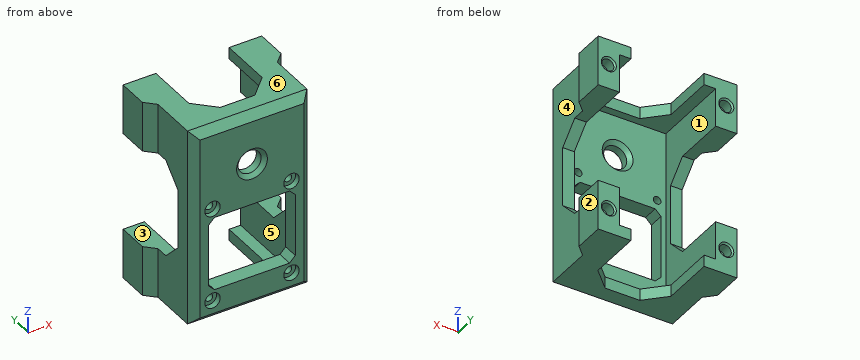
```python
from build123d import *

# Parameters (mm, degrees)
SKETCH1_W                                  = 25
SKETCH1_H                                  = 45.5
BOSS_EXTRUDE1_DEPTH                        = 4
SKETCH2_R                                  = 1
CUT_EXTRUDE1_DEPTH                         = 27.264281829
SKETCH3_W                                  = 22.5
SKETCH3_H                                  = 19.25
CUT_EXTRUDE2_DEPTH                         = 4
CHAMFER1_SIZE                              = 1.5
SKETCH4_R                                  = 3
CUT_EXTRUDE3_DEPTH                         = 27.264281829
SKETCH11_W                                 = 31
SKETCH11_H                                 = 51.5
SKETCH11_W_2                               = 25
SKETCH11_H_2                               = 45.5
BOSS_EXTRUDE5_DEPTH                        = 6
BOSS_EXTRUDE6_DEPTH                        = 18.75
SKETCH14_W                                 = 5.5
SKETCH14_H                                 = 13
BOSS_EXTRUDE7_DEPTH                        = 8
SKETCH15_R                                 = 1.55
CUT_EXTRUDE5_DEPTH                         = 3
MIRROR2_AT_THE_SECOND_PLANE_COPY_1_DEPTH   = 18.75
MIRROR2_AT_THE_SECOND_PLANE_COPY_2_SKETC_W = 5.5
MIRROR2_AT_THE_SECOND_PLANE_COPY_2_SKETC_H = 13
MIRROR2_AT_THE_SECOND_PLANE_COPY_2_DEPTH   = 8
MIRROR2_AT_THE_SECOND_PLANE_COPY_3_SKETC_R = 1.55
MIRROR2_AT_THE_SECOND_PLANE_COPY_3_DEPTH   = 3
CHAMFER3_SIZE                              = 2.5
CHAMFER4_SIZE                              = 5
CHAMFER5_SIZE                              = 2
SKETCH16_R                                 = 2
CUT_EXTRUDE6_DEPTH                         = 1.5
CHAMFER6_SIZE                              = 1
CHAMFER7_SIZE                              = 0.4
SKETCH17_R                                 = 1
CUT_EXTRUDE7_DEPTH                         = 4


with BuildPart() as part:
    # Sketch1 → Boss-Extrude1 (new body)
    with BuildSketch(Plane(origin=(0, 0, 0), x_dir=(1, 0, 0), z_dir=(0, 1, 0))):
        Rectangle(SKETCH1_W, SKETCH1_H)
    extrude(amount=BOSS_EXTRUDE1_DEPTH)

    # Sketch2 → Cut-Extrude1 (cut, through all)
    with BuildSketch(Plane(origin=(0, 4, 0), x_dir=(1, 0, 0), z_dir=(0, 1, 0))):
        with Locations(Location((-10.25, 20.25, 0), (0, 0, 270))):
            Circle(SKETCH2_R)
        with Locations(Location((10.25, 20.25, 0), (0, 0, 270))):
            Circle(SKETCH2_R)
        with Locations(Location((10.25, -4.2, 0), (0, 0, 270))):
            Circle(SKETCH2_R)
        with Locations(Location((-10.25, -4.2, 0), (0, 0, 270))):
            Circle(SKETCH2_R)
    extrude(amount=-CUT_EXTRUDE1_DEPTH, mode=Mode.SUBTRACT)

    # Sketch3 → Cut-Extrude2 (cut)
    with BuildSketch(Plane(origin=(0, 4, 0), x_dir=(1, 0, 0), z_dir=(0, 1, 0))):
        with Locations((0, 7.875)):
            Rectangle(SKETCH3_W, SKETCH3_H)
    extrude(amount=-CUT_EXTRUDE2_DEPTH, mode=Mode.SUBTRACT)

    # Chamfer1
    chamfer1_edges = [part.edges().sort_by_distance(p)[0] for p in [
        (11.25, 2, -17.5),
        (11.25, 2, 1.75),
        (-11.25, 2, 1.75),
        (-11.25, 2, -17.5),
    ]]
    chamfer(chamfer1_edges, length=CHAMFER1_SIZE)

    # Sketch4 → Cut-Extrude3 (cut, through all)
    with BuildSketch(Plane(origin=(0, 4, 0), x_dir=(1, 0, 0), z_dir=(0, 1, 0))):
        with Locations(Location((0, -12.5, 0), (0, 0, 270))):
            Circle(SKETCH4_R)
    extrude(amount=-CUT_EXTRUDE3_DEPTH, mode=Mode.SUBTRACT)

    # Sketch11 → Boss-Extrude5 (add)
    with BuildSketch(Plane.XZ):
        Rectangle(SKETCH11_W, SKETCH11_H)
        Rectangle(SKETCH11_W_2, SKETCH11_H_2, mode=Mode.SUBTRACT)
    extrude(amount=-BOSS_EXTRUDE5_DEPTH)

    # Sketch12 → Boss-Extrude6 (add)
    with BuildSketch(Plane(origin=(0, 6, 0), x_dir=(1, 0, 0), z_dir=(0, 1, 0))):
        Polygon((-15.5, 25.75), (-9.5, 25.75), (-9.5, 22.75), (-12.5, 22.75), (-12.5, 12.75), (-15.5, 12.75), align=None)
    boss_extrude6 = extrude(amount=BOSS_EXTRUDE6_DEPTH)

    # Sketch14 → Boss-Extrude7 (add)
    with BuildSketch(Plane(origin=(0, 24.75, 0), x_dir=(1, 0, 0), z_dir=(0, 1, 0))):
        with Locations((-15.25, 19.25)):
            Rectangle(SKETCH14_W, SKETCH14_H)
    boss_extrude7 = extrude(amount=-BOSS_EXTRUDE7_DEPTH)

    # Sketch15 → Cut-Extrude5 (cut)
    with BuildSketch(Plane(origin=(0, 24.75, 0), x_dir=(1, 0, 0), z_dir=(0, 1, 0))):
        with Locations(Location((-15.25, 19.25, 0), (0, 0, 270))):
            Circle(SKETCH15_R)
    cut_extrude5 = extrude(amount=-CUT_EXTRUDE5_DEPTH, mode=Mode.SUBTRACT)

    # Mirror2: Boss-Extrude6, Boss-Extrude7, Cut-Extrude5 across plane
    add(boss_extrude6.mirror(Plane(origin=(0, 0, 0), x_dir=(0, 0, 1), z_dir=(1, 0, 0))))
    add(boss_extrude7.mirror(Plane(origin=(0, 0, 0), x_dir=(0, 0, 1), z_dir=(1, 0, 0))))
    add(cut_extrude5.mirror(Plane(origin=(0, 0, 0), x_dir=(0, 0, 1), z_dir=(1, 0, 0))), mode=Mode.SUBTRACT)

    # Mirror2 at the second plane: Boss-Extrude6, Boss-Extrude7, Cut-Extrude5 across plane
    add(boss_extrude6.mirror(Plane.XY))
    add(boss_extrude7.mirror(Plane.XY))
    add(cut_extrude5.mirror(Plane.XY), mode=Mode.SUBTRACT)

    # Mirror2 at the second plane copy 1 sketc → Mirror2 at the second plane copy 1 (add)
    with BuildSketch(Plane(origin=(0, 6, 0), x_dir=(-1, 0, 0), z_dir=(0, 1, 0))):
        Polygon((-15.5, 25.75), (-9.5, 25.75), (-9.5, 22.75), (-12.5, 22.75), (-12.5, 12.75), (-15.5, 12.75), align=None)
    extrude(amount=MIRROR2_AT_THE_SECOND_PLANE_COPY_1_DEPTH)

    # Mirror2 at the second plane copy 2 sketc → Mirror2 at the second plane copy 2 (add)
    with BuildSketch(Plane(origin=(0, 24.75, 0), x_dir=(-1, 0, 0), z_dir=(0, 1, 0))):
        with Locations((-15.25, 19.25)):
            Rectangle(MIRROR2_AT_THE_SECOND_PLANE_COPY_2_SKETC_W, MIRROR2_AT_THE_SECOND_PLANE_COPY_2_SKETC_H)
    extrude(amount=-MIRROR2_AT_THE_SECOND_PLANE_COPY_2_DEPTH)

    # Mirror2 at the second plane copy 3 sketc → Mirror2 at the second plane copy 3 (cut)
    with BuildSketch(Plane(origin=(0, 24.75, 0), x_dir=(-1, 0, 0), z_dir=(0, 1, 0))):
        with Locations(Location((-15.25, 19.25, 0), (0, 0, 270))):
            Circle(MIRROR2_AT_THE_SECOND_PLANE_COPY_3_SKETC_R)
    extrude(amount=-MIRROR2_AT_THE_SECOND_PLANE_COPY_3_DEPTH, mode=Mode.SUBTRACT)

    # Chamfer3
    # the kernel refuses this chamfer: 2.5 mm, written as the material it adds along each edge
    with BuildSketch(Plane(origin=(-15.5, 16.75, -12.75), x_dir=(0.027495876610586317, -0.9996219169112968, 0), z_dir=(0, 0, -1))) as chamfer3_piece_1_section:
        Polygon((CHAMFER3_SIZE * 0.999621916911, CHAMFER3_SIZE * 0.0274958766106), (-CHAMFER3_SIZE * 0.0274958766106, CHAMFER3_SIZE * 0.999621916911), (0, 0), align=None)
    chamfer3_piece_1 = extrude(amount=13, mode=Mode.PRIVATE)
    chamfer3_piece_1 = split(chamfer3_piece_1, bisect_by=Plane(origin=(-18, 15.923989614, -19.25), z_dir=(1, 0, 0)), keep=Keep.TOP, mode=Mode.PRIVATE)
    add(chamfer3_piece_1)
    with BuildSketch(Plane(origin=(-15.5, 16.75, 12.75), x_dir=(0.027495876610586317, -0.9996219169112968, 0), z_dir=(0, 0, 1))) as chamfer3_piece_2_section:
        Polygon((CHAMFER3_SIZE * 0.999621916911, -CHAMFER3_SIZE * 0.0274958766106), (-CHAMFER3_SIZE * 0.0274958766106, -CHAMFER3_SIZE * 0.999621916911), (0, 0), align=None)
    chamfer3_piece_2 = extrude(amount=13, mode=Mode.PRIVATE)
    chamfer3_piece_2 = split(chamfer3_piece_2, bisect_by=Plane(origin=(-18, 15.923989614, 19.25), z_dir=(1, 0, 0)), keep=Keep.TOP, mode=Mode.PRIVATE)
    add(chamfer3_piece_2)
    with BuildSketch(Plane(origin=(15.5, 16.75, -12.75), x_dir=(-0.027495876610586317, -0.9996219169112968, 0), z_dir=(0, 0, -1))) as chamfer3_piece_3_section:
        Polygon((CHAMFER3_SIZE * 0.999621916911, -CHAMFER3_SIZE * 0.0274958766106), (-CHAMFER3_SIZE * 0.0274958766106, -CHAMFER3_SIZE * 0.999621916911), (0, 0), align=None)
    chamfer3_piece_3 = extrude(amount=13, mode=Mode.PRIVATE)
    chamfer3_piece_3 = split(chamfer3_piece_3, bisect_by=Plane(origin=(18, 15.923989614, -19.25), z_dir=(-1, 0, 0)), keep=Keep.TOP, mode=Mode.PRIVATE)
    add(chamfer3_piece_3)
    with BuildSketch(Plane(origin=(15.5, 16.75, 12.75), x_dir=(-0.027495876610586317, -0.9996219169112968, 0), z_dir=(0, 0, 1))) as chamfer3_piece_4_section:
        Polygon((CHAMFER3_SIZE * 0.999621916911, CHAMFER3_SIZE * 0.0274958766106), (-CHAMFER3_SIZE * 0.0274958766106, CHAMFER3_SIZE * 0.999621916911), (0, 0), align=None)
    chamfer3_piece_4 = extrude(amount=13, mode=Mode.PRIVATE)
    chamfer3_piece_4 = split(chamfer3_piece_4, bisect_by=Plane(origin=(18, 15.923989614, 19.25), z_dir=(-1, 0, 0)), keep=Keep.TOP, mode=Mode.PRIVATE)
    add(chamfer3_piece_4)

    # Chamfer4
    chamfer4_edges = [part.edges().sort_by_distance(p)[0] for p in [
        (-14, 6, -12.75),
        (-9.5, 6, -24.25),
        (-14, 6, 12.75),
        (-9.5, 6, 24.25),
        (14, 6, -12.75),
        (9.5, 6, -24.25),
        (14, 6, 12.75),
        (9.5, 6, 24.25),
    ]]
    chamfer(chamfer4_edges, length=CHAMFER4_SIZE)

    # Chamfer5
    chamfer5_edges = [part.edges().sort_by_distance(p)[0] for p in [
        (0, 0, -25.75),
        (15.5, 0, 0),
        (0, 0, 25.75),
        (-15.5, 0, 0),
    ]]
    chamfer(chamfer5_edges, length=CHAMFER5_SIZE)

    # Sketch16 → Cut-Extrude6 (cut)
    with BuildSketch(Plane.XZ):
        with Locations(Location((-10.25, 4.2, 0), (0, 0, 270))):
            Circle(SKETCH16_R)
        with Locations(Location((10.25, 4.2, 0), (0, 0, 270))):
            Circle(SKETCH16_R)
        with Locations(Location((10.25, -20.25, 0), (0, 0, 270))):
            Circle(SKETCH16_R)
        with Locations(Location((-10.25, -20.25, 0), (0, 0, 270))):
            Circle(SKETCH16_R)
    extrude(amount=-CUT_EXTRUDE6_DEPTH, mode=Mode.SUBTRACT)

    # Chamfer6
    chamfer6_edges = [part.edges().sort_by_distance(p)[0] for p in [
        (0, 0, 9.5),
        (0, 4, 9.5),
    ]]
    chamfer(chamfer6_edges, length=CHAMFER6_SIZE)

    # Chamfer7
    chamfer7_edges = [part.edges().sort_by_distance(p)[0] for p in [
        (-15.25, 24.75, -20.8),
        (-15.25, 24.75, 20.8),
        (15.25, 24.75, -20.8),
        (15.25, 24.75, 20.8),
    ]]
    chamfer(chamfer7_edges, length=CHAMFER7_SIZE)

    # Sketch17 → Cut-Extrude7 (cut)
    with BuildSketch(Plane(origin=(0, 21.75, 0), x_dir=(1, 0, 0), z_dir=(0, 1, 0))):
        with Locations(Location((-15.25, 19.25, 0), (0, 0, 270))):
            Circle(SKETCH17_R)
        with Locations(Location((15.25, 19.25, 0), (0, 0, 270))):
            Circle(SKETCH17_R)
        with Locations(Location((15.25, -19.25, 0), (0, 0, 270))):
            Circle(SKETCH17_R)
        with Locations(Location((-15.25, -19.25, 0), (0, 0, 270))):
            Circle(SKETCH17_R)
    extrude(amount=-CUT_EXTRUDE7_DEPTH, mode=Mode.SUBTRACT)


solid = part.part
```
The model under review builds one solid part; all positions refer to its coordinate system, in mm. Face numbers are marked on the shaded views. A direction names the side the tool comes from. Give positions to 0.01 mm unless a question says otherwise; leave off trailing zeros. Order: outer loops, then holes, each group sorted by start corner. A loop starts at its lowest first (then second) coordinate and runs counter-clockwise, first axis right, second up. Notation, with made-up numbers: (47, -1.75) - (65, -1.75) arc R31 ccw to (65, 37.25) - close; hole circle Ø11 at (-5.75, -38). An arc over 180 degrees is marked (long way). Use CSV: the item, a comma, the result in double quotes. Start each with the question number.
Q1. We need section D-D, the plane z = 4.2. Write out the cut boundary in (x, y), and give its area (3 significant figures).
Q2. Tool access review of the marked faces 1, 2 and 3: name each direction out of +Z, -Z, +X, -X, +Y, -Y from which nothing blocks a thin tool from reaching the whole face with its end or side.
Q3. We need section C-C, the plane y = 13.5. Write out the cut boundary in (x, z), and give its area (3 significant figures).
Q4. To check wall thickness, follow line 1 along X through (y, z) = (20.15, 19.25); line 2 along X through (y, z) = (3.35, 4.2); line 3 along Z through (x, y) = (-10, 8.5). State the ranges of each line that lie inside material, in increasing order. Write a range as [from, to].
Q5. We need section B-B, the plane z = -11. Write out the cut boundary in (x, y), and give its area (3 significant figures).
Q6. We need section A-A, the plane y = 18.5. Write out the cut boundary in (x, z).
Q7. Clearance check with flat-ended pins moving along their axes: pin 1 Ø1.2 at (x, z) = (-15.25, 19.25) entering from -Y; pin 2 Ø6 at (y, z) = (4.5, -10) entering from -X; pin 3 Ø1.9 at (x, z) = (-15.25, 19.25) entering from -Y. State where each tip first meets the part, or that it passes through.
Q8. The part is to be moulded in two halves that separate along X. For the marked faces 4, 5 and 6, say which applies: +X half, -X half, draft (parallel to the pull), parting line (faces both ways), or undercut.
Outcome:
1,outline,"(-15.5, 2) - (-13.5, 0) - (-12.25, 0) - (-12.25, 1.5) - (-11.25, 1.5) - (-11.25, 4) - (-12.5, 4) - (-12.5, 6) - (-15.5, 6) - close; (-9.25, 1.5) - (-8.25, 1.5) - (-8.25, 0) - (8.25, 0) - (8.25, 1.5) - (9.25, 1.5) - (9.25, 4) - (-9.25, 4) - close; (11.25, 1.5) - (12.25, 1.5) - (12.25, 0) - (13.5, 0) - (15.5, 2) - (15.5, 6) - (12.5, 6) - (12.5, 4) - (11.25, 4) - close"
1,area,"110 mm^2"
2,face 1,"+Y"
2,face 2,"+Z, -Z, +X, +Y, -Y"
2,face 3,"+X, -X, +Y"
3,outline,"(-15.5, -25.75) - (-9.5, -25.75) - (-9.5, -22.75) - (-12.5, -22.75) - (-12.5, -12.75) - (-15.5, -12.75) - close; (-15.5, 12.75) - (-12.5, 12.75) - (-12.5, 22.75) - (-9.5, 22.75) - (-9.5, 25.75) - (-15.5, 25.75) - close; (9.5, -25.75) - (15.5, -25.75) - (15.5, -12.75) - (12.5, -12.75) - (12.5, -22.75) - (9.5, -22.75) - close; (9.5, 22.75) - (12.5, 22.75) - (12.5, 12.75) - (15.5, 12.75) - (15.5, 25.75) - (9.5, 25.75) - close"
3,area,"192 mm^2"
4,line 1,"x = [-18, -16.25], [-14.25, -12.5], [12.5, 14.25], [16.25, 18]"
4,line 2,"x = [-15.5, -11.25], [-9.25, 9.25], [11.25, 15.5]"
4,line 3,"z = [-25.75, -22.75], [22.75, 25.75]"
5,outline,"(-15.5, 2) - (-13.5, 0) - (-11.25, 0) - (-11.25, 4) - (-12.5, 4) - (-12.5, 9.25) - (-15.5, 9.25) - close; (11.25, 0) - (13.5, 0) - (15.5, 2) - (15.5, 9.25) - (12.5, 9.25) - (12.5, 4) - (11.25, 4) - close"
5,area,"61.5 mm^2"
6,outline,"(-18, -25.75) - (-9.5, -25.75) - (-9.5, -22.75) - (-12.5, -22.75) - (-12.5, -12.75) - (-18, -12.75) - close; (-18, 12.75) - (-12.5, 12.75) - (-12.5, 22.75) - (-9.5, 22.75) - (-9.5, 25.75) - (-18, 25.75) - close; (9.5, -25.75) - (18, -25.75) - (18, -12.75) - (12.5, -12.75) - (12.5, -22.75) - (9.5, -22.75) - close; (9.5, 22.75) - (12.5, 22.75) - (12.5, 12.75) - (18, 12.75) - (18, 25.75) - (9.5, 25.75) - close; hole circle Ø2 at (-15.25, -19.25); hole circle Ø2 at (-15.25, 19.25); hole circle Ø2 at (15.25, -19.25); hole circle Ø2 at (15.25, 19.25)"
7,pin 1,"stops at y = 1.15"
7,pin 2,"stops at x = -15.5"
7,pin 3,"stops at y = 0.8"
8,face 4,"+X half"
8,face 5,"undercut"
8,face 6,"draft"
